Check sheet for the modelled part. Datum: model origin and axes. Units: mm. A direction names the side the tool comes from. Coordinates: 2 decimals unless noted, no trailing zeros. Loops run counter-clockwise (first coordinate to the right, second up) from the corner with the lowest first, then second, coordinate; pieces in that order, holes last. Notation, with made-up numbers: (64.25, 78) -> (76.25, 78) arc R18 cw to (76.25, 83) -> close; hole circle Ø4 at (-37.75, 79.25). An arc over 180 degrees is marked (long way). Use CSV: the item, a comma, the result in double quotes.
Autodesk Inventor part; units mm, degrees
ref_plane "YZ Plane" through (0, 0, 0) normal (1, 0, 0) x (0, 1, 0)
ref_plane "XZ Plane" through (0, 0, 0) normal (0, 1, 0) x (-1, 0, 0)
ref_plane "XY Plane" through (0, 0, 0) normal (0, 0, 1) x (1, 0, 0)
sketch "Esboço1" plane through (0, 0, 0) normal (0, 1, 0) x (-1, 0, 0)
  circle A0 centre (0, 0) radius 3.31
  circle A1 centre (0, 0) radius 14
  dimension "d2" = 6.62
  dimension "d3" = 28
extrude "Extrusão1" add sketch "Esboço1" along normal blind 60
sketch "Esboço2" plane through (0, 60, 0) normal (0, 1, 0) x (1, 0, 0)
  circle A0 centre (0, 0) radius 6.25
  dimension "d7" = 12.5
extrude "Extrusão2" cut sketch "Esboço2" against normal blind 9
sketch "Esboço3" plane through (0, 0, 0) normal (0, -1, 0) x (1, 0, 0)
  circle A0 centre (0, 0) radius 3.31
extrude "Extrusão3" add sketch "Esboço3" against normal blind 30
fillet "Arredondamento1" radius 1 5 edges at (14, 60, 0) (-6.25, 60, 0) (-6.25, 51, 0) (3.31, 51, 0) (3.31, 30, 0)
properties part number "peça encaixe telhado"
1) Cross-section at D-D on y = 35.5. Record the boundary of the cut face in (x, z).
Answer below:
outline,"circle Ø28 at (0, 0); hole circle Ø6.62 at (0, 0)"
2) Go/stop test with flat-tipped pins: pin 1 Ø1 at (x, y) = (-3, 31) entering from -Z (3 decimals); pin 2 Ø1.4 at (x, z) = (0.5, 0.5) entering from +Y; pin 3 Ø8.5 at (x, z) = (-1, -2) entering from +Y. Record where each tip stops, or that it passes through.
Answer below:
pin 1,"stops at z = -13.775"
pin 2,"stops at y = 30"
pin 3,"stops at y = 59.65"
3) Draft check along X on faces 3 (the cylindrical face through (-12.932, 29.087, 5.362)), 4 (the flat face through (-6, 60, -6)), 5 (the flat face through (0, 30, 0)). Enter one of: released by +X, released by -X, zero draft, split by the parting line, or undercut.
Answer below:
face 3,"split by the parting line"
face 4,"zero draft"
face 5,"undercut"
4) Cross-section at C-C on y = 6.5. Record the boundary of the cut face in (x, z), and give its area (3 significant figures).
Answer below:
outline,"circle Ø28 at (0, 0)"
area,"616 mm²"
5) Access from +Z, -Z, +X, -X, +Y, -Y to the whole of each face (thin tool, end or side, straight path). Record for faces 1 (the cylindrical face through (0.43, 40.37, -3.28)), 2 (the flat face through (0, 0, 0)).
Answer below:
face 1,"+Y"
face 2,"+Z, -Z, +X, -X, -Y"
6) Cross-section at A-A on x = 0. Record the boundary of the cut face in (y, z), and give its area (3 significant figures).
Answer below:
outline,"(0, -14) -> (59, -14) arc R1 ccw to (60, -13) -> (60, -7.25) arc R1 ccw to (59, -6.25) -> (52, -6.25) arc R1 cw to (51, -5.25) -> (51, -4.31) arc R1 ccw to (50, -3.31) -> (31, -3.31) arc R1 cw to (30, -2.31) -> (30, 2.31) arc R1 cw to (31, 3.31) -> (50, 3.31) arc R1 ccw to (51, 4.31) -> (51, 5.25) arc R1 cw to (52, 6.25) -> (59, 6.25) arc R1 ccw to (60, 7.25) -> (60, 13) arc R1 ccw to (59, 14) -> (0, 14) -> close"
area,"1,430 mm²"
7) Thickness scan on line 1 along Z through (x, y) = (0, 57); line 2 along Z through (x, y) = (0, 39.25); line 3 along X through (y, z) = (34, -0.25). Record the ranges inside material, lowest first. Write a range as from..to.
Answer below:
line 1,"z = -14..-6.25, 6.25..14"
line 2,"z = -14..-3.31, 3.31..14"
line 3,"x = -14..-3.3, 3.3..14"
8) Cross-section at B-B on z = 0. Record the boundary of the cut face in (x, y).
Answer below:
outline,"(-14, 0) -> (14, 0) -> (14, 59) arc R1 ccw to (13, 60) -> (7.25, 60) arc R1 ccw to (6.25, 59) -> (6.25, 52) arc R1 cw to (5.25, 51) -> (4.31, 51) arc R1 ccw to (3.31, 50) -> (3.31, 31) arc R1 cw to (2.31, 30) -> (-2.31, 30) arc R1 cw to (-3.31, 31) -> (-3.31, 50) arc R1 ccw to (-4.31, 51) -> (-5.25, 51) arc R1 cw to (-6.25, 52) -> (-6.25, 59) arc R1 ccw to (-7.25, 60) -> (-13, 60) arc R1 ccw to (-14, 59) -> close"
